Here's how the part is built. I have some questions about the finished solid (model axes, mm). A direction names the side the tool comes from. Give positions to 0.01 mm unless a question says otherwise; leave off trailing zeros. Write each loop counter-clockwise with the first axis right and the second up, starting at its lowest first coordinate (ties: lowest second). Pieces come first, ordered by that corner, then holes. Notation, with made-up numbers: (33, 4) - (81, 4) arc R15 cw to (81, 14) - close; hole circle Ø9 at (76, 8). An arc over 180 degrees is marked (long way). One line per item, written item: value. Start each with the question number.
1) Please list where these lines run through material, in increasing order: L1, parallel to Y at x = 102, z = 12.5; L2, parallel to X at y = 0.25, z = 11; L3, parallel to X at y = 0.5, z = -2. Write a range as [from, to].
2) We'd pull the mould along X, two halves only. Please class faces 1 (the flat face through (68, 0, 21.26)), 2 (the flat face through (79.096, 7, 9)), 3 (the flat face through (0, 0, 9)): +X half, -X half, draft (parallel to the pull), parting line (faces both ways), or undercut.
3) Imagine slicing it at C-C on x = 17. Write out the boundary of the cut face in (y, z), plus the area to 3 significant figures.
4) Imagine slicing it at B-B on y = 1.5. Write out the boundary of the cut face in (x, z).
5) On a 3-axis mill with a long thin cutter (end or side, diameter ignored), from which of +Z, -Z, +X, -X, +Y, -Y can I reach the whole of each face in a straight line? I mean faces 4 (the cylindrical face through (108.113, -6.715, -0.219)), 5 (the flat face through (126, -7.62, 12)), 6 (the flat face through (85, 9, -3.632)). Say none if no direction works.
6) Imagine slicing it at D-D on x = 137. Write out the boundary of the cut face in (y, z).
7) I'm going to push flat-ended pins straight in: P1, Ø4, axis at x = 122, y = 4.5, coming from the +Z side; P2, Ø4, axis at y = -11, z = 4.5, coming from the -X side; P3, Ø10, axis at x = 60, y = 9.5, coming from the +Z side; P4, Ø4.5, axis at y = 2.5, z = 29, coming from the -X side. Where does each tip first touch, or does it pass through?
from build123d import *

# Parameters (mm, degrees)
F1_DEPTH  = 173
F3_DEPTH  = 173.001
F5_DEPTH  = 173.001
F6_W      = 159.538
F6_H      = 15.24
F7_DEPTH  = 23.6865
F9_DEPTH  = 18.161
F11_DEPTH = 24.893
F13_DEPTH = 24.893


with BuildPart() as f1:
    # F0 (on Right) → F1 (new body)
    with BuildSketch(Plane.YZ):
        with BuildLine():
            ThreePointArc((-16, 0), (0, -6.2), (16, 0))
            Line((16, 0), (16, 22.539117))
            ThreePointArc((16, 22.539117), (15.933845, 22.979673), (15.741214, 23.381369))
            Line((15.741214, 23.381369), (6.946329, 36.342252))
            ThreePointArc((6.946329, 36.342252), (6.407476, 36.825401), (5.705115, 37))
            Line((5.705115, 37), (-5.705115, 37))
            ThreePointArc((-5.705115, 37), (-6.407476, 36.825401), (-6.946329, 36.342252))
            Line((-6.946329, 36.342252), (-15.741214, 23.381369))
            ThreePointArc((-15.741214, 23.381369), (-15.933845, 22.979673), (-16, 22.539117))
            Line((-16, 22.539117), (-16, 0))
        make_face()
    extrude(amount=F1_DEPTH)

    # F2 (on face) → F3 (cut, through all)
    with BuildSketch(Plane(origin=(0, 0, 0), x_dir=(0, -1, 0), z_dir=(-1, 0, 0))):
        Polygon((-16, 21.26), (-9.398, 21.26), (-9.398, 36.5), (9.398, 36.5), (9.398, 21.26), (16, 21.26), (16, 39.197723), (-16, 39.197723), align=None)
    extrude(amount=-F3_DEPTH, mode=Mode.SUBTRACT)

    # F4 (on face) → F5 (cut, through all)
    with BuildSketch(Plane(origin=(0, 0, 0), x_dir=(0, -1, 0), z_dir=(-1, 0, 0))):
        Polygon((-14.2875, 21.26), (-16, 21.26), (-16, -10.530328), (16, -10.530328), (16, 21.26), (14.2875, 21.26), (14.2875, -3.632), (-14.2875, -3.632), align=None)
    extrude(amount=-F5_DEPTH, mode=Mode.SUBTRACT)

    # F6 (on face) → F7 (cut, through all)
    with BuildSketch(Plane(origin=(0, 9.398, 0), x_dir=(-1, 0, 0), z_dir=(0, 1, 0))):
        with Locations((-79.769, 28.88)):
            Rectangle(F6_W, F6_H)
    extrude(amount=-F7_DEPTH, mode=Mode.SUBTRACT)

    # F8 (on face) → F9 (cut)
    with BuildSketch(Plane.XY.offset(21.26)):
        with BuildLine():
            Line((85.9796, -7.62), (151.918, -7.62))
            ThreePointArc((151.918, -7.62), (159.538, 0), (151.918, 7.62))
            Line((151.918, 7.62), (85.9796, 7.62))
            ThreePointArc((85.9796, 7.62), (78.3596, 0), (85.9796, -7.62))
        make_face()
    extrude(amount=-F9_DEPTH, mode=Mode.SUBTRACT)

    # F10 (on face) → F11 (cut, through all)
    with BuildSketch(Plane.XY.offset(21.26)):
        with BuildLine():
            Line((109.0682, -4.445), (109.0682, 4.445))
            ThreePointArc((109.0682, 4.445), (108.138264, 6.690064), (105.8932, 7.62))
            Line((105.8932, 7.62), (101.340681, 7.62))
            ThreePointArc((101.340681, 7.62), (99.723084, 8.189057), (98.0192, 8.382))
            Line((98.0192, 8.382), (79.8582, 8.382))
            Line((79.8582, 8.382), (79.8582, 5))
            Line((79.8582, 5), (75.7942, 5))
            Line((75.7942, 5), (75.7942, -1.642426))
            ThreePointArc((75.7942, -1.642426), (76.219569, -3.229926), (77.3817, -4.392056))
            Line((77.3817, -4.392056), (79.101182, -5.3848))
            ThreePointArc((79.101182, -5.3848), (80.089903, -7.51407), (82.2712, -8.382))
            Line((82.2712, -8.382), (98.0192, -8.382))
            ThreePointArc((98.0192, -8.382), (99.723084, -8.189057), (101.340681, -7.62))
            Line((101.340681, -7.62), (105.8932, -7.62))
            ThreePointArc((105.8932, -7.62), (108.138264, -6.690064), (109.0682, -4.445))
        make_face()
    extrude(amount=-F11_DEPTH, mode=Mode.SUBTRACT)

    # F12 (on face) → F13 (cut, through all)
    with BuildSketch(Plane.XY.offset(21.26)):
        Polygon((75.3116, -5.1765), (87.6052, -5.1765), (87.6052, 8.7071), (79.0962, 8.7071), (79.0962, 5.1765), (75.3116, 5.1765), align=None)
    extrude(amount=-F13_DEPTH, mode=Mode.SUBTRACT)


solid = f1.part
Numbers:
1. L1: [-14.29, -7.62], [7.62, 14.29]
1. L2: [0, 75.31], [159.53, 173]
1. L3: [0, 75.31], [109.07, 173]
2. face 1: draft
2. face 2: undercut
2. face 3: -X half
3. outline: (-14.29, -1.42) arc R23.75 ccw to (-10.74, -3.63) - (10.74, -3.63) arc R23.75 ccw to (14.29, -1.42) - (14.29, 21.26) - (-14.29, 21.26) - close
3. area: 704 mm^2
4. outline: (0, -3.63) - (75.31, -3.63) - (75.31, 21.26) - (0, 21.26) - close; (109.07, -3.63) - (173, -3.63) - (173, 36.5) - (159.54, 36.5) - (159.54, 21.26) - (159.39, 21.26) - (159.39, 3.1) - (109.07, 3.1) - close
5. face 4: +Z, -Z
5. face 5: +Z
5. face 6: -Z, +X, -X, +Y, -Y
6. outline: (-14.29, -1.42) arc R23.75 ccw to (-10.74, -3.63) - (10.74, -3.63) arc R23.75 ccw to (14.29, -1.42) - (14.29, 21.26) - (7.62, 21.26) - (7.62, 3.1) - (-7.62, 3.1) - (-7.62, 21.26) - (-14.29, 21.26) - close
7. P1: z = 3.1
7. P2: x = 0
7. P3: z = 21.26
7. P4: x = 159.54
